Autodesk Inventor part; units mm, degrees
ref_plane "YZ Plane" through (0, 0, 0) normal (1, 0, 0) x (0, 1, 0)
ref_plane "XZ Plane" through (0, 0, 0) normal (0, 1, 0) x (-1, 0, 0)
ref_plane "XY Plane" through (0, 0, 0) normal (0, 0, 1) x (1, 0, 0)
sketch "Sketch1" plane through (0, 0, 0) normal (0, 0, 1) x (1, 0, 0)
  line L0 (6.5024, 17.6276) -> (-6.5024, 17.6276)
  line L1 (-6.5024, 12.5476) -> (6.5024, 12.5476) construction
  line L2 (6.5024, 12.5476) -> (13.7468, 0)
  line L3 (6.5024, 12.5476) -> (20.9911, 12.5476) construction
  line L4 (-6.5024, 12.5476) -> (0.742, 0)
  line L5 (-6.5024, 12.5476) -> (7.9863, 12.5476) construction
  line L6 (0, 12.5476) -> (7.2444, 0) construction
  line L7 (0, 12.5476) -> (14.4887, 12.5476) construction
  circle A0 centre (7.2444, 0) radius 2.1844
  circle A1 centre (7.2444, 0) radius 3.7719
  circle A2 centre (7.2444, 0) radius 6.5024 construction
  arc A3 (0.742, 0) -> (13.7468, 0) centre (7.2444, 3.7542) ccw
  line L8 (-6.5024, 17.6276) -> (-6.5024, 12.5476)
  line L9 (6.5024, 17.6276) -> (6.5024, 12.5476)
  point P0 (0, 0)
  dimension "d11" = 17.6276
  dimension "d37" = 5.08
  dimension "d38" = 60
  dimension "d39" = 60
  dimension "d40" = 60
  dimension "d41" = 4.3688
  dimension "d42" = 7.5438
  dimension "d43" = 13.0048
extrude "Extrusion1" add sketch "Sketch1" along normal blind 20.32 contours L9 L2 A3 A1 L4 L8 L0 | A3 A1 | A0 picked at (10.4509, 0.2998)
sketch "Sketch3" plane through (-6.5024, 17.6276, 0) normal (0, 1, 0) x (1, 0, 0)
  line L0 (6.6548, -14.4145) -> (6.6548, -20.32) construction
  line L1 (13.0048, 0) -> (0, 0) construction
  line L2 (6.5024, 0) -> (6.5024, -20.32) construction
  line L3 (13.0048, -20.32) -> (0, -20.32) construction
  line L4 (13.0048, 0) -> (13.0048, -20.32) construction
  line L5 (13.0048, -10.16) -> (0, -10.16) construction
  line L6 (0, 0) -> (0, -20.32) construction
  circle A0 centre (6.5024, -10.16) radius 1.9685 construction
  point P0 (6.5024, 0)
  dimension "d21" = 6.5024
  dimension "d22" = 10.16
  dimension "d23" = 3.937
hole "Hole1" at (0, 17.6276, 10.16) direction (0, -1, 0) diameter 3.937 end through all
sketch "Sketch7" plane through (-6.5024, 12.5476, 0) normal (-1, 0, 0) x (0, 0, 1)
  line L0 (0, 5.08) -> (20.32, 5.08) construction
  line L1 (10.16, 5.08) -> (10.16, -16.3018) construction
  line L2 (0, -16.3018) -> (20.32, -16.3018) construction
  line L3 (0, 0) -> (20.32, 0)
  line L4 (10.16, 0) -> (15.494, 0)
  line L5 (10.16, 0) -> (4.826, 0)
  line L6 (4.826, 0) -> (4.826, -4.7752)
  line L7 (15.494, 0) -> (15.494, -4.7752)
  line L8 (10.16, -16.3018) -> (6.985, -16.3018)
  line L9 (10.16, -16.3018) -> (13.335, -16.3018)
  line L10 (6.985, -16.3018) -> (6.985, -4.7752)
  line L11 (6.985, -4.7752) -> (4.826, -4.7752)
  line L12 (13.335, -16.3018) -> (13.335, -4.7752)
  line L13 (13.335, -4.7752) -> (15.494, -4.7752)
  point P0 (0, -12.5476)
  dimension "d47" = 5.334
  dimension "d48" = 5.334
  dimension "d49" = 4.7752
  dimension "d50" = 4.7752
  dimension "d51" = 3.175
  dimension "d52" = 3.175
extrude "Extrusion5" cut sketch "Sketch7" against normal through all
extrude "Extrusion6" cut sketch "Sketch1" along normal blind 2.54 contours A3 A1 | A1 A3 | A0
extrude "Extrusion7" cut sketch "Sketch1" along normal through all contours A0
sketch "Sketch8" plane through (0, 0, 20.32) normal (0, 0, 1) x (1, 0, 0)
  circle A0 centre (7.2444, 0) radius 2.1844 construction
  circle A1 centre (7.2444, 0) radius 4.2545 construction
  line L0 (11.4989, 0) -> (9.0425, -4.2545)
  line L1 (5.4462, -4.2545) -> (2.9899, 0)
  line L2 (2.9899, 0) -> (5.1171, 3.6845)
  line L3 (5.1171, 3.6845) -> (9.3716, 3.6845)
  line L4 (9.3716, 3.6845) -> (11.4989, 0)
  line L5 (5.4462, -4.2545) -> (9.0425, -4.2545)
  point P0 (0, 0)
  point P1 (9.3716, -3.6845)
  point P2 (5.1171, -3.6845)
  dimension "d59" = 8.509
extrude "Extrusion8" cut sketch "Sketch8" against normal blind 2.54
properties part number "omni wheel wheel holder tilted"
Here's how the part is built. I have some questions about the finished solid (model axes, mm). A direction names the side the tool comes from. Round coordinates to 2 decimals unless told otherwise and drop trailing zeros. Order: outer loops, then holes, each group sorted by start corner. A loop starts at its lowest first (then second) coordinate and runs counter-clockwise, first axis right, second up. Notation, with made-up numbers: (18, -19) -> (63, -19) arc R20 cw to (63, 10) -> close; hole circle Ø9 at (36, 23.5). An arc over 180 degrees is marked (long way). Return JSON: item names as keys, results as strings.
Q1. Which directions (+Z, -Z, +X, -X, +Y, -Y) give clear straight access to the entire face, cutting with the end or side of a thin tool? Please do faces 5 (the cylindrical face through (7.09, 3.77, 1.25)), 6 (the flat face through (1, 10, 4.826)), 7 (the flat face through (6.502, 15, 10)), 8 (the flat face through (4.04, 1.82, 19.07)), 9 (the flat face through (5, 3, 6.985)).
Filled sheet:
{"face 5": "-Z", "face 6": "+X, -X", "face 7": "+Z, -Z, +X, +Y", "face 8": "+Z", "face 9": "+X, -X, -Y"}
Q2. I need wall thicknesses on line 1 along Z through (x, y) = (7.5, 8.5); line 2 along Z through (x, y) = (12.5, -1.25) (3 decimals); line 3 along X through (y, z) = (14.75, 14.25). Which ranges of each line are inside material? Lowest first, please. Write a range as from..to.
Filled sheet:
{"line 1": "z = 0..4.83, 15.49..20.32", "line 2": "z = 0..6.985, 13.335..20.32", "line 3": "x = -6.5..6.5"}
Q3. If we section it at D-D on y = 9.5: List the corners of the cut face in (x, z) for me.
Filled sheet:
{"outline": "(-4.74, 0) -> (8.26, 0) -> (8.26, 4.83) -> (-4.74, 4.83) -> close; (-4.74, 15.49) -> (8.26, 15.49) -> (8.26, 20.32) -> (-4.74, 20.32) -> close"}
Q4. For pin 1 Ø4 at (x, y) = (10.5, 14) entering from +Z; pin 2 Ø5.5 at (x, z) = (-2, 10.5) entering from -Y; pin 3 Ø1.3 at (x, z) = (7.5, 19) entering from -Y; pin 4 Ø5 at (y, z) = (2.5, 14) entering from -X, each with a flat end and sliding along its axis, tell me the tip position at first contact or that it passes through.
Filled sheet:
{"pin 1": "passes through", "pin 2": "stops at y = 12.55", "pin 3": "stops at y = 3.68", "pin 4": "stops at x = -2.14"}
Q5. If we section it at A-A on z = 10.16: List the corners of the cut face in (x, y) for me, plus the area to 3 significant figures.
Filled sheet:
{"outline": "(-6.5, 12.55) -> (-1.97, 12.55) -> (-1.97, 17.63) -> (-6.5, 17.63) -> close; (1.97, 12.55) -> (6.5, 12.55) -> (6.5, 17.63) -> (1.97, 17.63) -> close", "area": "46.1 mm^2"}
Q6. If we mould it in two halves opening along X, with no side actions, what happens to faces 1 (the flat face through (1, 9, 0)), 2 (the flat face through (-2.93, 6.36, 16.78)), 3 (the flat face through (9, -2, 2.54)), 4 (the cylindrical face through (6.96, -2.166, 4.731))? For each: released by +X, released by -X, zero draft, split by the parting line, or undercut.
Filled sheet:
{"face 1": "zero draft", "face 2": "released by -X", "face 3": "undercut", "face 4": "undercut"}
Q7. If we section it at C-C on y = 16.25: List the corners of the cut face in (x, z) for me, plus the area to 3 significant figures.
Filled sheet:
{"outline": "(-6.5, 0) -> (6.5, 0) -> (6.5, 20.32) -> (-6.5, 20.32) -> close; hole circle Ø3.94 at (0, 10.16)", "area": "252 mm^2"}
Q8. If we section it at B-B on x = -1.5: List the corners of the cut face in (y, z) for me (3 decimals).
Filled sheet:
{"outline": "(3.883, 0) -> (17.628, 0) -> (17.628, 8.885) -> (12.548, 8.885) -> (12.548, 4.826) -> (7.772, 4.826) -> (7.772, 6.985) -> (3.883, 6.985) -> close; (3.883, 13.335) -> (7.772, 13.335) -> (7.772, 15.494) -> (12.548, 15.494) -> (12.548, 11.435) -> (17.628, 11.435) -> (17.628, 20.32) -> (3.883, 20.32) -> close"}
